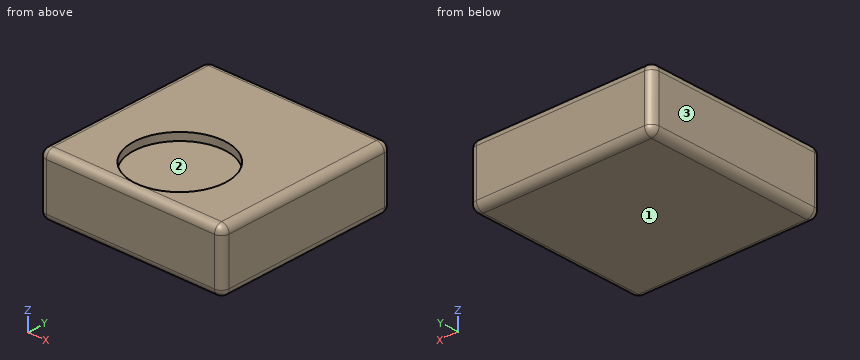
```python
from build123d import *

# Parameters (mm, degrees)
SKETCH1_W           = 152.4
SKETCH1_H           = 152.4
BOSS_EXTRUDE1_DEPTH = 25.4
SKETCH2_R           = 38.1
CUT_EXTRUDE1_DEPTH  = 6.35
FILLET1_R           = 6.35


with BuildPart() as part:
    # Sketch1 → Boss-Extrude1 (new, symmetric)
    with BuildSketch(Plane.XY):
        Rectangle(SKETCH1_W, SKETCH1_H)
    extrude(amount=BOSS_EXTRUDE1_DEPTH, both=True)

    # Sketch2 → Cut-Extrude1 (cut)
    with BuildSketch(Plane.XY.offset(25.4)):
        with Locations((0, -31.75)):
            Circle(SKETCH2_R)
    extrude(amount=-CUT_EXTRUDE1_DEPTH, mode=Mode.SUBTRACT)

    # Fillet1
    fillet1_edges = [part.edges().sort_by_distance(p)[0] for p in [
        (-76.2, 0, 25.4),
        (0, -76.2, 25.4),
        (76.2, 0, 25.4),
        (0, -76.2, -25.4),
        (-76.2, 0, -25.4),
        (0, 76.2, -25.4),
        (76.2, 0, -25.4),
        (76.2, -76.2, 0),
        (-76.2, -76.2, 0),
        (-76.2, 76.2, 0),
        (76.2, 76.2, 0),
        (0, 76.2, 25.4),
    ]]
    fillet(fillet1_edges, radius=FILLET1_R - 0.0001)  # a hair under: the kernel refuses the full size


solid = part.part
```
Read the model definition and answer for the solid it produces. Units are mm, in the model's axes. Face numbers are marked on the shaded views. Coordinates: 2 decimals unless noted, no trailing zeros. Order: outer loops, then holes, each group sorted by start corner. A loop starts at its lowest first (then second) coordinate and runs counter-clockwise, first axis right, second up. Notation, with made-up numbers: (48.25, 88) - (66.25, 88) arc R28 ccw to (66.25, 127) - close; hole circle Ø6 at (55, 47). An arc over 180 degrees is marked (long way). Answer as a JSON object with one key per item and string values. Group by question number.
Item 1: Consider probe 1 along Y at (x, z) = (0, 20.5); probe 2 along Z at (x, y) = (2, -25); probe 3 along X at (y, z) = (-31, 24). Determine where each line is inside the solid, lowest interval first. Write a range as from..to.
Item 2: A flat-ended cylindrical pin translates along its axis: P1, Ø10, axis at x = 2, y = -16, coming from the +Z side. Find the tip coordinate at first contact, or state that the pin passes through.
Item 3: Section C-C (z = 22) is taken. Give the vertices of the cut face in (x, y), plus the area to 3 significant figures.
Item 4: Section A-A (y = -31.75) is taken. Give the vertices of the cut face in (x, z), plus the area to 3 significant figures.
Item 5: The mould has two halves that part along X. Classify the marked faces 1, 2 and 3: +X half, -X half, draft (parallel to the pull), parting line (faces both ways), or undercut.
Results are:
{
 "1": {"probe 1": "y = -76.03..-69.85, 6.35..76.03", "probe 2": "z = -25.4..19.05", "probe 3": "x = -73.83..-38.09, 38.09..73.83"},
 "2": {"P1": "stops at z = 19.05"},
 "3": {"outline": "(-75.47, -69.85) arc R5.62 ccw to (-69.85, -75.47) - (69.85, -75.47) arc R5.62 ccw to (75.47, -69.85) - (75.47, 69.85) arc R5.62 ccw to (69.85, 75.47) - (-69.85, 75.47) arc R5.62 ccw to (-75.47, 69.85) - close; hole circle Ø76.2 at (0, -31.75)", "area": "18,200 mm^2"},
 "4": {"outline": "(-76.2, -19.05) arc R6.35 ccw to (-69.85, -25.4) - (69.85, -25.4) arc R6.35 ccw to (76.2, -19.05) - (76.2, 19.05) arc R6.35 ccw to (69.85, 25.4) - (38.1, 25.4) - (38.1, 19.05) - (-38.1, 19.05) - (-38.1, 25.4) - (-69.85, 25.4) arc R6.35 ccw to (-76.2, 19.05) - close", "area": "7,220 mm^2"},
 "5": {"face 1": "draft", "face 2": "undercut", "face 3": "-X half"}
}
